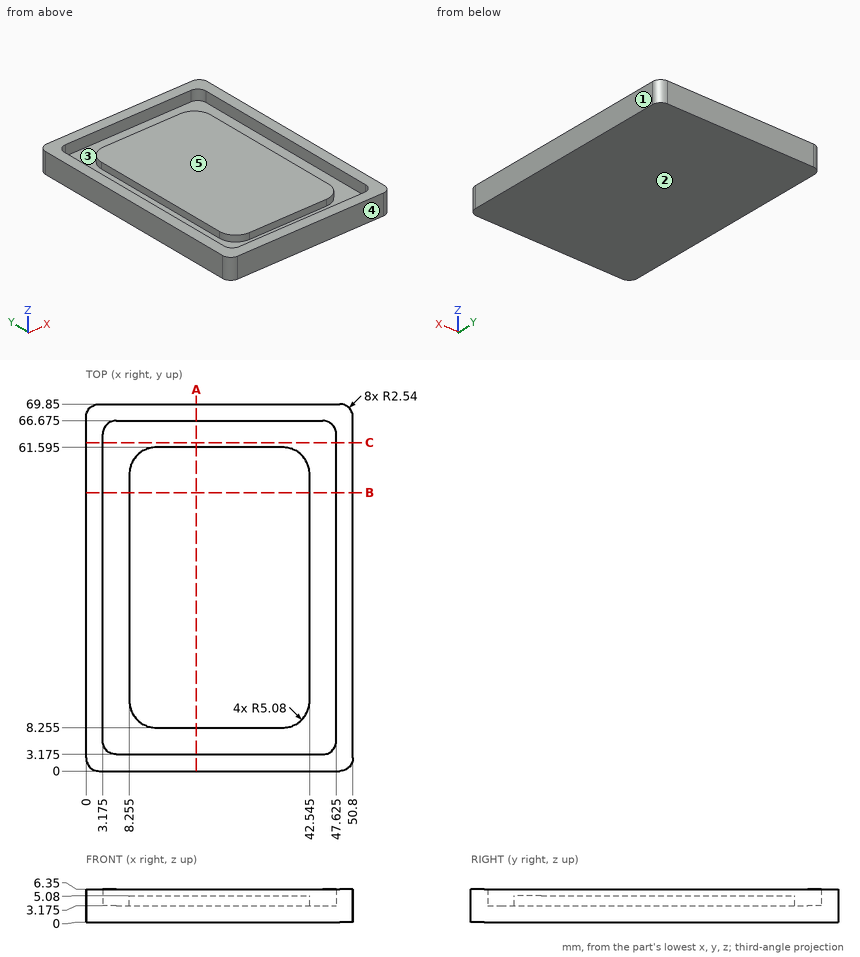
Source: three-view drawing plus pictorial views. Frame: mm from the lowest corner of the part. A direction names the side the tool comes from. Round coordinates to 2 decimals unless told otherwise and drop trailing zeros. Write each loop counter-clockwise with the first axis right and the second up, starting at its lowest first coordinate (ties: lowest second). Pieces come first, ordered by that corner, then holes. Notation, with made-up numbers: M 67,-27 L 100,-27 A17 ccw 100,5 Z; hole C -6,-22 d9. An arc over 180 degrees is marked long. One line per item, written item: value. Start each with the question number.
Item 1: Pin query (flat end, axial travel): pin 1 (5 mm diameter, centred on x = 40.5, y = 33, fed in from +Z). Return the tip coordinate at first contact, or that it passes through.
Item 2: Section query B-B (y = 53). Return the cut outline in (x, z) (3 decimals).
Item 3: Section query C-C (y = 62.5). Return the cut outline in (x, z) (3 decimals).
Item 4: Ray query, L1, parallel to Y at x = 23, z = 3.25 (3 decimals); L2, parallel to X at y = 56, z = 4.75 (3 decimals); L3, parallel to Y at x = 44.5, z = 6.25 (3 decimals). Return the intervals inside material, ascending. Write a range as from..to.
Item 5: Mould query, pull axis X, two halves, no side actions, for the marked faces 1, 2 and 3. Classes: pulls with the +X half, pulls with the -X half, needs draft (parallel to the pull), parting line crosses it, or undercut.
Item 6: Set-up query: the marked faces 4 and 5. Return all of +Z, -Z, +X, -X, +Y, -Y with unobstructed straight access to the full face (end or side cutting, diameter ignored); none if empty.
Item 7: Section query A-A (x = 21). Return the cut outline in (y, z) (3 decimals), plus the area to 3 significant figures.
Result set:
1. pin 1: stops at z = 5.08
2. outline: M 0,0 L 50.8,0 L 50.8,6.35 L 47.625,6.35 L 47.625,3.175 L 42.545,3.175 L 42.545,5.08 L 8.255,5.08 L 8.255,3.175 L 3.175,3.175 L 3.175,6.35 L 0,6.35 Z
3. outline: M 0,0 L 50.8,0 L 50.8,6.35 L 47.625,6.35 L 47.625,3.175 L 3.175,3.175 L 3.175,6.35 L 0,6.35 Z
4. L1: y = 0..3.175, 8.255..61.595, 66.675..69.85
4. L2: x = 0..3.175, 8.255..42.545, 47.625..50.8
4. L3: y = 0..3.175, 66.675..69.85
5. face 1: pulls with the +X half
5. face 2: needs draft
5. face 3: undercut
6. face 4: +Z, -Z, +X, -X, -Y
6. face 5: +Z
7. outline: M 0,0 L 69.85,0 L 69.85,6.35 L 66.675,6.35 L 66.675,3.175 L 61.595,3.175 L 61.595,5.08 L 8.255,5.08 L 8.255,3.175 L 3.175,3.175 L 3.175,6.35 L 0,6.35 Z
7. area: 344 mm²
